Read the model definition and answer for the solid it produces. Units are mm, in the model's axes. Face numbers are marked on the shaded views. A direction names the side the tool comes from. Round coordinates to 2 decimals unless told otherwise and drop trailing zeros. Loops run counter-clockwise (first coordinate to the right, second up) from the corner with the lowest first, then second, coordinate; pieces in that order, holes last. Notation, with made-up numbers: M -14.5,-21.5 L 19.5,-21.5 A4 ccw 19.5,-17.5 Z; hole C -11,-22 d11. An arc over 180 degrees is marked long. Write each question's results on one line, items separated by ' | '.
from build123d import *

# Parameters (mm, degrees)
SKETCH_1_R               = 100
EXTRUDE_1_DEPTH          = 20
SKETCH_2_W               = 173
SKETCH_2_H               = 150
CUT_EXTRUDE_1_DEPTH      = 15
SKETCH_3_R               = 2.5
CUT_EXTRUDE_2_DEPTH      = 143.214626533
PATTERN_CIRCULAR_2_COUNT = 12
SKETCH_4_W               = 45
SKETCH_4_H               = 25
CUT_EXTRUDE_3_DEPTH      = 143.828568571


with BuildPart() as part:
    # Sketch 1 → Extrude 1 (new body)
    with BuildSketch(Plane(origin=(0, 0, 0), x_dir=(1, 0, 0), z_dir=(0, 1, 0))):
        with Locations(Location((0, 0, 0), (0, 0, 270))):
            Circle(SKETCH_1_R)
    extrude(amount=EXTRUDE_1_DEPTH)

    # Sketch 2 → Cut-Extrude 1 (cut)
    with BuildSketch(Plane(origin=(0, 20, 0), x_dir=(1, 0, 0), z_dir=(0, 1, 0))):
        Rectangle(SKETCH_2_W, SKETCH_2_H)
    extrude(amount=-CUT_EXTRUDE_1_DEPTH, mode=Mode.SUBTRACT)

    # Sketch 3 → Cut-Extrude 2 (cut, through all)
    with BuildSketch(Plane(origin=(0, 5, 0), x_dir=(1, 0, 0), z_dir=(0, 1, 0))):
        with Locations(Location((0, 65, 0), (0, 0, 270))):
            Circle(SKETCH_3_R)
        with Locations(Location((0, 55, 0), (0, 0, 270))):
            Circle(SKETCH_3_R)
        with Locations(Location((0, 45, 0), (0, 0, 270))):
            Circle(SKETCH_3_R)
        with Locations(Location((0, 35, 0), (0, 0, 270))):
            Circle(SKETCH_3_R)
        with Locations(Location((0, 25, 0), (0, 0, 270))):
            Circle(SKETCH_3_R)
        with Locations(Location((0, 15, 0), (0, 0, 270))):
            Circle(SKETCH_3_R)
    cut_extrude_2 = extrude(amount=-CUT_EXTRUDE_2_DEPTH, mode=Mode.SUBTRACT)

    # Pattern Circular 2: Cut-Extrude 2 ×12 about axis
    pattern_circular_2_axis = Axis((0, 0, 0), (0, 1, 0))
    for i in range(1, PATTERN_CIRCULAR_2_COUNT):
        add(cut_extrude_2.rotate(pattern_circular_2_axis, i * 360 / PATTERN_CIRCULAR_2_COUNT), mode=Mode.SUBTRACT)

    # Sketch 4 → Cut-Extrude 3 (cut, through all)
    with BuildSketch(Plane(origin=(0, 20, 0), x_dir=(1, 0, 0), z_dir=(0, 1, 0))):
        with Locations((0, -87.5)):
            Rectangle(SKETCH_4_W, SKETCH_4_H)
    extrude(amount=-CUT_EXTRUDE_3_DEPTH, mode=Mode.SUBTRACT)


solid = part.part
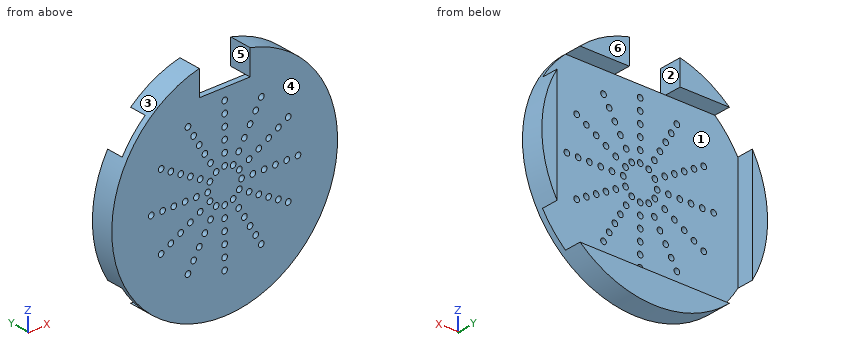
Item 1: The mould has two halves that part along X. Classify the marked faces 1, 2, 3 and 4: pulls with the +X half, pulls with the -X half, needs draft (parallel to the pull), parting line crosses it, or undercut.
Outcome:
face 1: undercut | face 2: undercut | face 3: parting line crosses it | face 4: needs draft
Item 2: The part is cut by section C-C (z = -80.5). Determine the outline of the cut face in (x, y), plus the area to 3 significant figures.
Outcome:
outline: M -59.33,0 L 59.33,0 L 59.33,20 L -59.33,20 Z | area: 2,370 mm2
Item 3: Straight lines are drawn through the part: line 1 (Y direction, x = 19.5, z = 8.5); line 2 (X direction, y = 2.75, z = -34.5); line 3 (X direction, y = 6, z = 38). For each, find the intervals that lie inside material, in ascending order.
Outcome:
line 1: y = 0 to 5 | line 2: x = -93.86 to -57.79, -54.79 to -2.45, 2.45 to 54.79, 57.79 to 93.86 | line 3: x = -92.5 to -86.5, 86.5 to 92.5
Item 4: Flat-ended cylindrical pins translate along their axes: pin 1 (8 mm diameter, centred on x = 47.63, z = -27.5, fed in from +Y); pin 2 (1 mm diameter, centred on x = -39, y = 15, fed in from -Z); pin 3 (6 mm diameter, centred on y = 6.5, z = 44, fed in from +X); pin 4 (4.5 mm diameter, centred on x = -47.63, z = -27.5, fed in from -Y). Find the tip coordinate at first contact, or state that the pin passes through.
Outcome:
pin 1: stops at y = 5 | pin 2: stops at z = -92.29 | pin 3: stops at x = 91.21 | pin 4: passes through
Item 5: The part is cut by section A-A (y = 17.5). Determine the outline of the cut face in (x, z).
Outcome:
outline: M -86.5,-50.18 L -86.5,50.18 A100 ccw Z; M -66.14,-75 A100 ccw 66.14,-75 Z; M -66.14,75 L -22.5,75 L -22.5,97.44 A100 ccw Z; M 22.5,75 L 66.14,75 A100 ccw 22.5,97.44 Z; M 86.5,-50.18 A100 ccw 86.5,50.18 Z
Item 6: The part is cut by section B-B (z = 84). Determine the outline of the cut face in (x, y).
Outcome:
outline: M -54.26,0 L -22.5,0 L -22.5,20 L -54.26,20 Z; M 22.5,0 L 54.26,0 L 54.26,20 L 22.5,20 Z
Item 7: For the marked faces 5 and 6, determine the directions among +Z, -Z, +X, -X, +Y, -Y from which every point of the face is accessible in a straight line to the end or side of a thin tool.
Outcome:
face 5: +Z, +Y, -Y | face 6: +Z, -Z, +X, -X, +Y
